Here's the drawing with two shaded views (mm, measured from the low corner). I have some questions. Round coordinates to 2 decimals unless told otherwise and drop trailing zeros. Order: outer loops, then holes, each group sorted by start corner. A loop starts at its lowest first (then second) coordinate and runs counter-clockwise, first axis right, second up. Notation, with made-up numbers: (-36, 55) - (-23, 55) arc R18 ccw to (-23, 68) - close; hole circle Ø8 at (8.5, 36). An arc over 180 degrees is marked (long way). One line per item, written item: value.
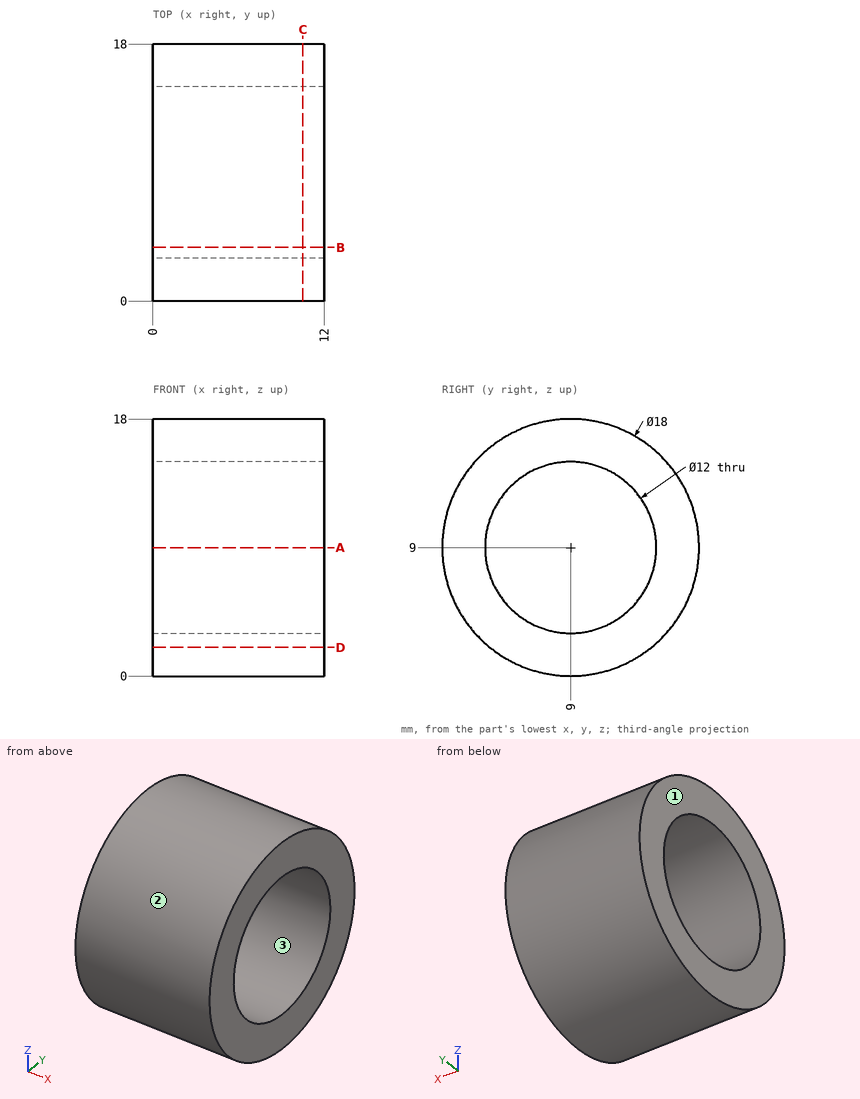
Q1. If we section it at B-B, the plane y = 3.75: Please give me the cut outline in (x, z), then the cut area to 3 significant figures.
Results list:
outline: (0, 1.69) - (12, 1.69) - (12, 6.1) - (0, 6.1) - close; (0, 11.9) - (12, 11.9) - (12, 16.31) - (0, 16.31) - close
area: 106 mm²
Q2. If we section it at A-A, the plane z = 9: Please give me the cut outline in (x, y), then the cut area to 3 significant figures.
Results list:
outline: (0, 0) - (12, 0) - (12, 3) - (0, 3) - close; (0, 15) - (12, 15) - (12, 18) - (0, 18) - close
area: 72.0 mm²
Q3. If we section it at D-D, the plane z = 2: Please give me the cut outline in (x, y).
Results list:
outline: (0, 3.34) - (12, 3.34) - (12, 14.66) - (0, 14.66) - close
Q4. We'd pull the mould along Y, two halves only. Please class the marked faces 1, 2 and 3: released by +Y, released by -Y, zero draft, split by the parting line, or undercut.
Results list:
face 1: zero draft
face 2: split by the parting line
face 3: undercut
Q5. If we section it at C-C, the plane x = 10.5: Please give me the cut outline in (y, z).
Results list:
outline: circle Ø18 at (9, 9); hole circle Ø12 at (9, 9)
Q6. Will these pins go through, and if not, where does the flat tip stop? pin 1 (1 mm diameter, centred on x = 8.5, y = 5, fed in from -Z); pin 2 (1.5 mm diameter, centred on x = 4.5, y = 6.5, fed in from +Z); pin 3 (5 mm diameter, centred on x = 9, y = 12, fed in from +Z); pin 4 (2 mm diameter, centred on y = 16, z = 3, fed in from +X).
Results list:
pin 1: z = 0.71
pin 2: z = 17.83
pin 3: z = 17.99
pin 4: x = 12
Q7. If I drill on line 1 along Y through (x, z) = (6.75, 9); line 2 along Z through (x, y) = (3, 6.75); line 3 along Z through (x, y) = (6.5, 8.5), over which ranges is the centre line in solid material (lowest first)?
Results list:
line 1: 0 to 3, 15 to 18
line 2: 0.29 to 3.44, 14.56 to 17.71
line 3: 0.01 to 3.02, 14.98 to 17.99
